Could you check a few things on this model? Use its own coordinates, in mm. A direction names the side the tool comes from. Coordinates: 2 decimals unless noted, no trailing zeros. Order: outer loops, then holes, each group sorted by start corner. A loop starts at its lowest first (then second) coordinate and runs counter-clockwise, first axis right, second up. Notation, with made-up numbers: (-20.5, -35) -> (11.5, -35) arc R19 ccw to (11.5, -1) -> close; hole circle Ø5 at (37.5, -6). An arc over 180 degrees is marked (long way). Put each result on its own line as item: value. Start each with the question number.
Q1. Please list where these lines run through material, in increasing order: line 1 along X through (y, z) = (110.5, 2.5); line 2 along Z through (x, y) = (-25.5, 151).
Q2. If we section it at D-D (y = -50.5): Please give me the cut outline in (x, z), and give its area (3 significant figures).
Q3. For faces 1 (the face through (25, -5, 0)), 2 (the face through (0, -325, 27)), which set-ups out of +Z, -Z, +X, -X, +Y, -Y let a thin tool reach every point of the face, with its end or its side?
Q4. If we section it at C-C (y = -230.5): Please give me the cut outline in (x, z).
Q5. If we section it at B-B (z = 15.5): Please give me the cut outline in (x, y).
Q6. We'd pull the mould along X, two halves only. Please class faces 3 (the face through (-30, -5, 0)), 4 (the face through (0, -5, 25)), 5 (the face through (30, -5, 0)): +X half, -X half, draft (parallel to the pull), parting line (faces both ways), or undercut.
Q7. If we section it at A-A (x = -14): Please give me the cut outline in (y, z), and give its area (3 significant figures).
Q8. Will these pins go through, and if not, where does the flat tip stop? pin 1 (4 mm diameter, centred on x = 13, z = -23.5, fed in from -Y); pin 2 (2.5 mm diameter, centred on x = -28, y = -294, fed in from -Z).
from build123d import *

# Parameters (mm, degrees)
F0_W     = 50
F0_H     = 50
F1_DEPTH = 325
F3_DEPTH = 60.001


# Not quite as in the source:
# - a feature names something its author has since deleted; it is built from what else it names


with BuildPart() as f1:
    # F0 (on Front) → F1 (new body, symmetric)
    with BuildSketch(Plane.XZ):
        with BuildLine():
            Line((-25, -30), (25, -30))
            ThreePointArc((25, -30), (28.5355339059, -28.5355339059), (30, -25))
            Line((30, -25), (30, 25))
            ThreePointArc((30, 25), (28.5355339059, 28.5355339059), (25, 30))
            Line((25, 30), (-25, 30))
            ThreePointArc((-25, 30), (-28.5355339059, 28.5355339059), (-30, 25))
            Line((-30, 25), (-30, -25))
            ThreePointArc((-30, -25), (-28.5355339059, -28.5355339059), (-25, -30))
        make_face()
        Rectangle(F0_W, F0_H, mode=Mode.SUBTRACT)
    extrude(amount=F1_DEPTH, both=True)

    # F2 (on face) → F3 (cut, through all)
    with BuildSketch(Plane.YZ.offset(30)):
        Polygon((-325, -5), (-347.579985857, -5), (-354.4286191463, -50.3063426539), (-215, -50.3063426539), (-215, -30), (-237, -25), (-325, -25), align=None)
        with BuildLine():
            Line((325, -25), (311.5831239518, -25))
            ThreePointArc((311.5831239518, -25), (303.6602540378, -28.7228132327), (295, -30))
            Line((295, -30), (295, -47.2164526592))
            Line((295, -47.2164526592), (357.106402663, -47.2164526592))
            Line((357.106402663, -47.2164526592), (357.106402663, 0))
            Line((357.106402663, 0), (325, 0))
            Line((325, 0), (325, -25))
        make_face()
        with BuildLine():
            ThreePointArc((325, 0), (321.4338203685, -14.1863716546), (311.5831239518, -25))
            Line((311.5831239518, -25), (325, -25))
            Line((325, -25), (325, 0))
        make_face()
    extrude(amount=-F3_DEPTH, mode=Mode.SUBTRACT)


solid = f1.part
The answers:
1. line 1: -30 to -25, 25 to 30
1. line 2: -29.97 to 29.97
2. outline: (-30, -25) arc R5 ccw to (-25, -30) -> (25, -30) arc R5 ccw to (30, -25) -> (30, 25) arc R5 ccw to (25, 30) -> (-25, 30) arc R5 ccw to (-30, 25) -> close; hole (-25, -25) -> (25, -25) -> (25, 25) -> (-25, 25) -> close
2. area: 1,080 mm^2
3. face 1: +Y, -Y
3. face 2: +Z, -Z, +X, -X, -Y
4. outline: (-30, -25) arc R5 ccw to (-29.78, -26.48) -> (29.78, -26.48) arc R5 ccw to (30, -25) -> (30, 25) arc R5 ccw to (25, 30) -> (-25, 30) arc R5 ccw to (-30, 25) -> close; hole (-25, -25) -> (25, -25) -> (25, 25) -> (-25, 25) -> close
5. outline: (-30, -325) -> (-25, -325) -> (-25, 325) -> (-30, 325) -> close; (25, -325) -> (30, -325) -> (30, 325) -> (25, 325) -> close
6. face 3: -X half
6. face 4: undercut
6. face 5: +X half
7. outline: (-325, 25) -> (325, 25) -> (325, 30) -> (-325, 30) -> close; (-237, -25) -> (-215, -30) -> (295, -30) arc R30 ccw to (311.58, -25) -> close
7. area: 5,910 mm^2
8. pin 1: y = -237
8. pin 2: z = -25
